```python
from build123d import *

# Parameters (mm, degrees)
F0_R     = 15
F0_R_2   = 11.25
F1_DEPTH = 2.5
F2_SIZE  = 0.5
F3_R     = 0.964531


with BuildPart() as f1:
    # F0 (on Top) → F1 (new body)
    with BuildSketch(Plane.XY):
        Circle(F0_R)
        Circle(F0_R_2, mode=Mode.SUBTRACT)
    extrude(amount=F1_DEPTH)

    # F2
    f2_edges = [f1.edges().sort_by_distance(p)[0] for p in [
        (-11.25, 0, 2.5),
    ]]
    chamfer(f2_edges, length=F2_SIZE)

    # F3
    f3_edges = [f1.edges().sort_by_distance(p)[0] for p in [
        (-15, 0, 2.5),
        (-15, 0, 0),
    ]]
    fillet(f3_edges, radius=F3_R)


solid = f1.part
```
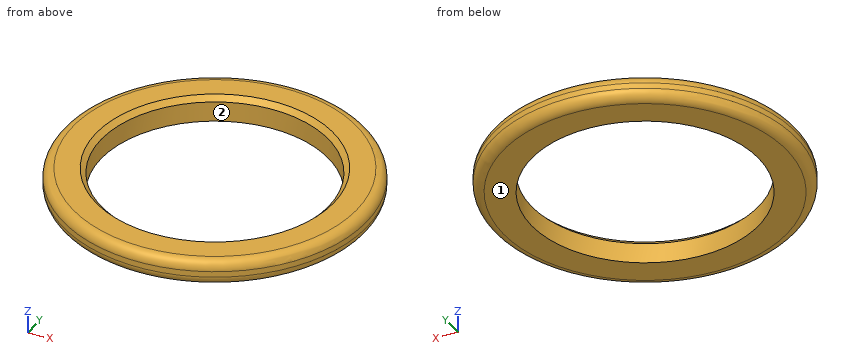
Could you check a few things on this model? Use its own coordinates, in mm. Face numbers are marked on the shaded views. Coordinates: 2 decimals unless noted, no trailing zeros. Write each loop counter-clockwise with the first axis right and the second up, starting at its lowest first coordinate (ties: lowest second). Pieces come first, ordered by that corner, then holes. Notation, with made-up numbers: (65, -11) -> (76, -11) arc R24 cw to (76, 15) -> close; hole circle Ø11 at (10.25, 64.5). An arc over 180 degrees is marked (long way). Return JSON: item names as keys, results as strings.
(1) I'm going to push a flat-ended pin straight in: pin 1 (1.5 mm diameter, centred on x = -9.5, z = 0.5, fed in from -Y). Where does the tip first touch, or does it pass through?
Numbers:
{"pin 1": "stops at y = -12.12"}
(2) Imagine slicing it at C-C, the plane z = 0.5. Please give me the cut outline in (x, y), then the cut area to 3 significant figures.
Numbers:
{"outline": "circle Ø29.76 at (0, 0); hole circle Ø22.5 at (0, 0)", "area": "298 mm2"}
(3) Imagine slicing it at A-A, the plane x = 0. Please give me the cut outline in (y, z), then the cut area to 3 significant figures.
Numbers:
{"outline": "(-15, 0.96) arc R0.96 ccw to (-14.04, 0) -> (-11.25, 0) -> (-11.25, 2) -> (-11.75, 2.5) -> (-14.04, 2.5) arc R0.96 ccw to (-15, 1.54) -> close; (11.25, 0) -> (14.04, 0) arc R0.96 ccw to (15, 0.96) -> (15, 1.54) arc R0.96 ccw to (14.04, 2.5) -> (11.75, 2.5) -> (11.25, 2) -> close", "area": "17.7 mm2"}
(4) We'd pull the mould along Y, two halves only. Please class the marked faces 1 and 2: +Y half, -Y half, draft (parallel to the pull), parting line (faces both ways), or undercut.
Numbers:
{"face 1": "draft", "face 2": "undercut"}
(5) I need wall thicknesses on L1, parallel to Y at x = 0, z = 1.3; L2, parallel to Y at x = -10, z = 0.4; L3, parallel to X at y = -2.75, z = 2.2. Which ranges of each line are inside material? Lowest first, please.
Numbers:
{"L1": "y = -15 to -11.25, 11.25 to 15", "L2": "y = -10.93 to -5.15, 5.15 to 10.93", "L3": "x = -14.48 to -11.11, 11.11 to 14.48"}
